Can you work these out from the model? Positions are in its coordinate system, mm. Face numbers are marked on the shaded views. A direction names the side the tool comes from. Give positions to 0.01 mm unless a question says otherwise; leave off trailing zeros. Write each loop counter-clockwise with the first axis right and the second up, starting at its lowest first coordinate (ties: lowest second). Pieces come first, ordered by that corner, then holes.
1. Thinking about a two-plate mould opening in X: for the marked faces 1, 2 and 3, which applies, pulls with the +X half, pulls with the -X half, needs draft (parallel to the pull), parting line crosses it, or undercut?
2. If I drill on probe 1 along Y at (x, z) = (16, 12); probe 2 along Y at (x, z) = (16, 7.75); probe 3 along X at (y, z) = (14.5, 13.75), over which ranges is the centre line in solid material (lowest first)?
3. On a 3-axis mill with a long thin cutter (end or side, diameter ignored), from which of +Z, -Z, +X, -X, +Y, -Y can I reach the whole of each face in a straight line? I mean the marked faces 4 and 5. Say none if no direction works.
4. I'm going to push flat-ended pins straight in: pin 1 (10 mm diameter, centred on x = 59.5, y = 18.5, fed in from +Z); pin 2 (1 mm diameter, centred on y = 55.5, z = 3.5, fed in from +X); pin 3 (1 mm diameter, centred on y = 12.5, z = 7.5, fed in from -X). Where does each tip first touch, or does it pass through?
5. Suppose I cut it at B-B (x = 18). Please give me the cut outline in (y, z), and give its area (3 significant figures).
6. Suppose I cut it at D-D (x = 60.5). Please give me the cut outline in (y, z), and give its area (3 significant figures).
7. Suppose I cut it at C-C (y = 50.5). Please give me the cut outline in (x, z).
8. Suppose I cut it at A-A (z = 15.75). Please give me the cut outline in (x, y).
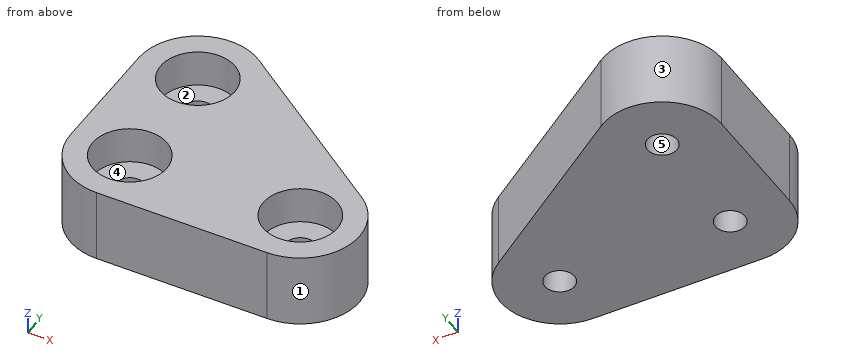
```python
from build123d import *

# Parameters (mm, degrees)
F0_R     = 10
F0_R_2   = 4
F1_DEPTH = 20
F2_R     = 10
F2_R_2   = 4
F3_DEPTH = 10


with BuildPart() as f1:
    # F0 (on Top) → F1 (new body)
    with BuildSketch(Plane.XY):
        with BuildLine():
            ThreePointArc((0, 16), (4.686292, 4.686292), (16, 0))
            Line((16, 0), (62.072559, 0))
            ThreePointArc((62.072559, 0), (77.309287, 11.117161), (71.37237, 29.019736))
            Line((71.37237, 29.019736), (25.299811, 61.928706))
            ThreePointArc((25.299811, 61.928706), (8.678695, 63.135653), (0, 48.908971))
            Line((0, 48.908971), (0, 16))
        make_face()
        with Locations((16, 16)):
            Circle(F0_R, mode=Mode.SUBTRACT)
        with Locations((62.072559, 16)):
            Circle(F0_R, mode=Mode.SUBTRACT)
        with Locations((16, 48.908971)):
            Circle(F0_R, mode=Mode.SUBTRACT)
        with Locations((16, 48.908971)):
            Circle(F0_R)
        with Locations((16, 48.908971)):
            Circle(F0_R_2, mode=Mode.SUBTRACT)
        with Locations((62.072559, 16)):
            Circle(F0_R)
        with Locations((62.072559, 16)):
            Circle(F0_R_2, mode=Mode.SUBTRACT)
        with Locations((16, 16)):
            Circle(F0_R)
        with Locations((16, 16)):
            Circle(F0_R_2, mode=Mode.SUBTRACT)
    extrude(amount=F1_DEPTH)

    # F2 (on face) → F3 (cut)
    with BuildSketch(Plane.XY.offset(20)):
        with Locations((16, 48.908971)):
            Circle(F2_R)
        with Locations((16, 48.908971)):
            Circle(F2_R_2, mode=Mode.SUBTRACT)
        with Locations((16, 16)):
            Circle(F2_R)
        with Locations((16, 16)):
            Circle(F2_R_2, mode=Mode.SUBTRACT)
        with Locations((62.072559, 16)):
            Circle(F2_R)
        with Locations((62.072559, 16)):
            Circle(F2_R_2, mode=Mode.SUBTRACT)
    extrude(amount=-F3_DEPTH, mode=Mode.SUBTRACT)


solid = f1.part
```
Checks:
1. face 1: pulls with the +X half
1. face 2: undercut
1. face 3: parting line crosses it
2. probe 1: y = 0 to 6, 26 to 38.91, 58.91 to 64.91
2. probe 2: y = 0 to 12, 20 to 44.91, 52.91 to 64.91
2. probe 3: x = 0.07 to 6.11, 25.89 to 52.19, 71.96 to 78
3. face 4: +Z
3. face 5: +Z, -Z
4. pin 1: stops at z = 10
4. pin 2: stops at x = 35
4. pin 3: stops at x = 0.28
5. outline: (0, 0) - (12.54, 0) - (12.54, 10) - (6.2, 10) - (6.2, 20) - (0, 20) - close; (19.46, 0) - (45.44, 0) - (45.44, 10) - (39.11, 10) - (39.11, 20) - (25.8, 20) - (25.8, 10) - (19.46, 10) - close; (52.37, 0) - (64.78, 0) - (64.78, 20) - (58.71, 20) - (58.71, 10) - (52.37, 10) - close
5. area: 765 mm2
6. outline: (0, 0) - (12.32, 0) - (12.32, 10) - (6.12, 10) - (6.12, 20) - (0, 20) - close; (19.68, 0) - (36.79, 0) - (36.79, 20) - (25.88, 20) - (25.88, 10) - (19.68, 10) - close
6. area: 465 mm2
7. outline: (0.08, 0) - (12.33, 0) - (12.33, 10) - (6.13, 10) - (6.13, 20) - (0.08, 20) - close; (19.67, 0) - (41.3, 0) - (41.3, 20) - (25.87, 20) - (25.87, 10) - (19.67, 10) - close
8. outline: (0, 16) arc R16 ccw to (16, 0) - (62.07, 0) arc R16 ccw to (71.37, 29.02) - (25.3, 61.93) arc R16 ccw to (0, 48.91) - close; hole circle Ø20 at (16, 16); hole circle Ø20 at (16, 48.91); hole circle Ø20 at (62.07, 16)
